from build123d import *

# Parameters (mm, degrees)
BOSS_EXTRUDE2_DEPTH = 12
SKETCH2_R           = 5
CUT_EXTRUDE1_DEPTH  = 29
SKETCH3_R           = 10
CUT_EXTRUDE3_DEPTH  = 1.5
SKETCH4_R           = 22
SKETCH4_R_2         = 12.5
BOSS_EXTRUDE3_DEPTH = 96
BOSS_EXTRUDE4_START = -76
BOSS_EXTRUDE4_DEPTH = 76
BOSS_EXTRUDE5_START = -57
BOSS_EXTRUDE5_DEPTH = 57
SKETCH7_W           = 16
SKETCH7_H           = 8
CUT_EXTRUDE4_DEPTH  = 50
SKETCH8_R           = 6
CUT_EXTRUDE5_DEPTH  = 20
SKETCH9_R           = 5
CUT_EXTRUDE7_DEPTH  = 28
FILLET1_R           = 5


with BuildPart() as part:
    # Sketch1 → Boss-Extrude2 (new body)
    with BuildSketch(Plane(origin=(0, 0, 0), x_dir=(1, 0, 0), z_dir=(0, 1, 0))):
        with BuildLine():
            Line((-32.5, 52.5), (32.5, 52.5))
            ThreePointArc((32.5, 52.5), (46.642135624, 46.642135624), (52.5, 32.5))
            Line((52.5, 32.5), (52.5, -32.5))
            ThreePointArc((52.5, -32.5), (46.642135624, -46.642135624), (32.5, -52.5))
            Line((32.5, -52.5), (-32.5, -52.5))
            ThreePointArc((-32.5, -52.5), (-46.642135624, -46.642135624), (-52.5, -32.5))
            Line((-52.5, -32.5), (-52.5, 32.5))
            ThreePointArc((-52.5, 32.5), (-46.642135624, 46.642135624), (-32.5, 52.5))
        make_face()
    extrude(amount=BOSS_EXTRUDE2_DEPTH)

    # Sketch2 → Cut-Extrude1 (cut)
    with BuildSketch(Plane(origin=(0, 12, 0), x_dir=(1, 0, 0), z_dir=(0, 1, 0))):
        with Locations(Location((-32.5, 32.5, 0), (0, 0, 270))):
            Circle(SKETCH2_R)
        with Locations(Location((32.5, 32.5, 0), (0, 0, 270))):
            Circle(SKETCH2_R)
        with Locations(Location((32.5, -32.5, 0), (0, 0, 270))):
            Circle(SKETCH2_R)
        with Locations(Location((-32.5, -32.5, 0), (0, 0, 270))):
            Circle(SKETCH2_R)
    extrude(amount=-CUT_EXTRUDE1_DEPTH, mode=Mode.SUBTRACT)

    # Sketch3 → Cut-Extrude3 (cut)
    with BuildSketch(Plane(origin=(0, 12, 0), x_dir=(1, 0, 0), z_dir=(0, 1, 0))):
        with Locations(Location((-32.5, 32.5, 0), (0, 0, 270))):
            Circle(SKETCH3_R)
        with Locations(Location((32.5, 32.5, 0), (0, 0, 90))):
            Circle(SKETCH3_R)
        with Locations(Location((-32.5, -32.5, 0), (0, 0, 90))):
            Circle(SKETCH3_R)
        with Locations(Location((32.5, -32.5, 0), (0, 0, 270))):
            Circle(SKETCH3_R)
    extrude(amount=-CUT_EXTRUDE3_DEPTH, mode=Mode.SUBTRACT)

    # Sketch4 → Boss-Extrude3 (add)
    with BuildSketch(Plane(origin=(0, 12, 0), x_dir=(1, 0, 0), z_dir=(0, 1, 0))):
        with Locations(Location((0, 0, 0), (0, 0, 270))):
            Circle(SKETCH4_R)
        with Locations(Location((0, 0, 0), (0, 0, 270))):
            Circle(SKETCH4_R_2, mode=Mode.SUBTRACT)
    extrude(amount=BOSS_EXTRUDE3_DEPTH)

    # Sketch5 → Boss-Extrude4 (add)
    with BuildSketch(Plane(origin=(0, 108, 0), x_dir=(1, 0, 0), z_dir=(0, 1, 0)).offset(BOSS_EXTRUDE4_START)):
        with BuildLine():
            Line((25, 15), (25, -15))
            Line((25, -15), (16.093476939, -15))
            ThreePointArc((16.093476939, -15), (22, 0), (16.093476939, 15))
            Line((16.093476939, 15), (25, 15))
        make_face()
    extrude(amount=BOSS_EXTRUDE4_DEPTH)

    # Sketch6 → Boss-Extrude5 (add)
    with BuildSketch(Plane(origin=(0, 108, 0), x_dir=(1, 0, 0), z_dir=(0, 1, 0)).offset(BOSS_EXTRUDE5_START)):
        with BuildLine():
            Line((8, 20.493901532), (8, 32))
            Line((8, 32), (-22, 32))
            Line((-22, 32), (-22, 0))
            ThreePointArc((-22, 0), (-12.409673646, 18.165902125), (8, 20.493901532))
        make_face()
    extrude(amount=BOSS_EXTRUDE5_DEPTH)

    # Sketch7 → Cut-Extrude4 (cut)
    with BuildSketch(Plane(origin=(0, 108, 0), x_dir=(1, 0, 0), z_dir=(0, 1, 0))):
        with Locations((-5, 21)):
            Rectangle(SKETCH7_W, SKETCH7_H)
    extrude(amount=-CUT_EXTRUDE4_DEPTH, mode=Mode.SUBTRACT)

    # Sketch8 → Cut-Extrude5 (cut)
    with BuildSketch(Plane(origin=(25, 0, 0), x_dir=(0, 0, -1), z_dir=(1, 0, 0))):
        with Locations((0, 88)):
            Circle(SKETCH8_R)
        with Locations((0, 58)):
            Circle(SKETCH8_R)
    extrude(amount=-CUT_EXTRUDE5_DEPTH, mode=Mode.SUBTRACT)

    # Sketch9 → Cut-Extrude7 (cut)
    with BuildSketch(Plane(origin=(0, 0, -32), x_dir=(-1, 0, 0), z_dir=(0, 0, -1))):
        with Locations(Location((7, 93, 0), (0, 0, 345.590947366))):
            Circle(SKETCH9_R)
        with Locations(Location((7, 71, 0), (0, 0, 345.590947366))):
            Circle(SKETCH9_R)
    extrude(amount=-CUT_EXTRUDE7_DEPTH, mode=Mode.SUBTRACT)

    # Fillet1
    fillet1_edges = [part.edges().sort_by_distance(p)[0] for p in [
        (0, 12, -22),
    ]]
    fillet(fillet1_edges, radius=FILLET1_R)


solid = part.part
Here's how the part is built. I have some questions about the finished solid (model axes, mm). A direction names the side the tool comes from. Round coordinates to 2 decimals unless told otherwise and drop trailing zeros. Loops run counter-clockwise (first coordinate to the right, second up) from the corner with the lowest first, then second, coordinate; pieces in that order, holes last. Notation, with made-up numbers: (-5, -12.5) -> (27, -12.5) arc R12 ccw to (27, 1.5) -> close; hole circle Ø8 at (-6, 20). An arc over 180 degrees is marked (long way). Write each question's results on one line, items separated by ' | '.
(1) If we section it at C-C, the plane z = 30.5: List the corners of the cut face in (x, y) for me.
Worked answers:
outline: (-52.5, 0) -> (-37.08, 0) -> (-37.08, 10.5) -> (-42.3, 10.5) -> (-42.3, 12) -> (-52.5, 12) -> close; (-27.92, 0) -> (27.92, 0) -> (27.92, 10.5) -> (22.7, 10.5) -> (22.7, 12) -> (-22.7, 12) -> (-22.7, 10.5) -> (-27.92, 10.5) -> close; (37.08, 0) -> (52.5, 0) -> (52.5, 12) -> (42.3, 12) -> (42.3, 10.5) -> (37.08, 10.5) -> close
(2) If we section it at A-A, the plane y = 8.5: List the corners of the cut face in (x, z) for me, then the cut area to 3 significant figures.
Worked answers:
outline: (-52.5, -32.5) arc R20 ccw to (-32.5, -52.5) -> (32.5, -52.5) arc R20 ccw to (52.5, -32.5) -> (52.5, 32.5) arc R20 ccw to (32.5, 52.5) -> (-32.5, 52.5) arc R20 ccw to (-52.5, 32.5) -> close; hole circle Ø10 at (-32.5, -32.5); hole circle Ø10 at (-32.5, 32.5); hole circle Ø10 at (32.5, -32.5); hole circle Ø10 at (32.5, 32.5) | area: 10,400 mm2
(3) If we section it at B-B, the plane y = 49.5: List the corners of the cut face in (x, z) for me.
Worked answers:
outline: (16.09, -15) -> (25, -15) -> (25, 15) -> (16.09, 15) arc R22 ccw (long way) to start; hole circle Ø25 at (0, 0)
(4) If we section it at D-D, the plane x = 44.5: List the corners of the cut face in (y, z) for me.
Worked answers:
outline: (0, -48.5) -> (12, -48.5) -> (12, 48.5) -> (0, 48.5) -> close
(5) We'd pull the mould along X, two halves only. Please class faces 1 (the face through (7, 108, -11)), 2 (the face through (-46.486, 5.916, 46.797)), 3 (the face through (34.9, 10.5, 27.9)), 4 (the face through (-5, 58, -21)): released by +X, released by -X, zero draft, split by the parting line, or undercut.
Worked answers:
face 1: zero draft | face 2: released by -X | face 3: undercut | face 4: undercut
(6) If I drill on L1, parallel to Y at x = -7, z = -29; L2, parallel to Y at x = 19.5, z = 0; L3, parallel to X at y = 3.5, z = 32.5, over which ranges is the centre line in solid material (lowest first)?
Worked answers:
L1: 0 to 12, 51 to 66, 76 to 88, 98 to 108 | L2: 0 to 52, 64 to 82, 94 to 108 | L3: -52.5 to -37.5, -27.5 to 27.5, 37.5 to 52.5
(7) For P1, Ø1.5, axis at x = 37.5, z = 34, coming from the +Y side; P2, Ø9, axis at x = -7, y = 71, coming from the +Z side; P3, Ø8, axis at x = -8, y = 94, coming from the +Z side; P4, Ø9, axis at x = -32.5, z = 32.5, coming from the +Y side, each with a flat end and sliding along its axis, tell me the tip position at first contact or that it passes through.
Worked answers:
P1: y = 10.5 | P2: z = 21.86 | P3: z = 21.63 | P4: through
(8) For faces 5 (the face through (18, 88, 6)), 6 (the face through (-7, 79, -32)), 7 (the face through (3, 83, -21)), 8 (the face through (25, 69, 0)), which set-ups out of +Z, -Z, +X, -X, +Y, -Y let a thin tool reach every point of the face, with its end or its side?
Worked answers:
face 5: +X | face 6: -Z, +X, -X, +Y | face 7: +Y | face 8: +Z, -Z, +X, +Y
